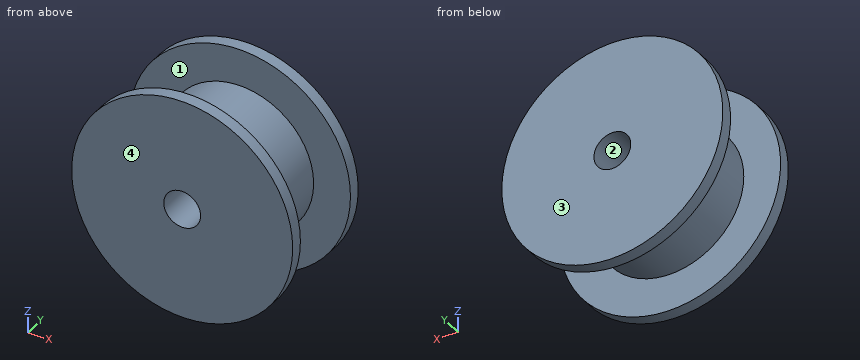
from build123d import *

# Parameters (mm, degrees)
SKETCH_1_R          = 9
EXTRUDE_1_DEPTH     = 1
SKETCH_2_R          = 6
EXTRUDE_2_DEPTH     = 6.5
SKETCH_3_R          = 9
EXTRUDE_3_DEPTH     = 1
SKETCH_4_R          = 1.5
CUT_EXTRUDE_1_DEPTH = 9.5


with BuildPart() as part:
    # 草图1 → 凸台-拉伸1 (new body)
    with BuildSketch(Plane(origin=(0, 0, 0), x_dir=(1, 0, 0), z_dir=(0, 1, 0))):
        Circle(SKETCH_1_R)
    extrude(amount=EXTRUDE_1_DEPTH)

    # 草图2 → 凸台-拉伸2 (add)
    with BuildSketch(Plane(origin=(0, 1, 0), x_dir=(1, 0, 0), z_dir=(0, 1, 0))):
        Circle(SKETCH_2_R)
    extrude(amount=EXTRUDE_2_DEPTH)

    # 草图3 → 凸台-拉伸3 (add)
    with BuildSketch(Plane(origin=(0, 7.5, 0), x_dir=(1, 0, 0), z_dir=(0, 1, 0))):
        Circle(SKETCH_3_R)
    extrude(amount=EXTRUDE_3_DEPTH)

    # 草图4 → 切除-拉伸1 (cut, through all)
    with BuildSketch(Plane(origin=(0, 8.5, 0), x_dir=(1, 0, 0), z_dir=(0, 1, 0))):
        Circle(SKETCH_4_R)
    extrude(amount=-CUT_EXTRUDE_1_DEPTH, mode=Mode.SUBTRACT)


solid = part.part
Can you work these out from the model? Positions are in its coordinate system, mm. Face numbers are marked on the shaded views. Coordinates: 2 decimals unless noted, no trailing zeros. Loops run counter-clockwise (first coordinate to the right, second up) from the corner with the lowest first, then second, coordinate; pieces in that order, holes last. Notation, with made-up numbers: M 52.25,82 L 111.25,82 A18 ccw 111.25,116 Z; hole C 38,-22.5 d10. An arc over 180 degrees is marked long. Answer as CSV lines item,"result". Start each with the question number.
1. If I drill on probe 1 along Z at (x, y) = (0, 3.75); probe 2 along Y at (x, z) = (-7, 4.75), over which ranges is the centre line in solid material (lowest first)? Write a range as [from, to].
2. Suppose I cut it at A-A, the plane x = 0. List the corners of the cut face in (y, z) for me.
3. For pin 1 Ø1 at (x, y) = (3, 4) entering from -Z, with a flat end and sliding along its axis, tell me the tip position at first contact or that it passes through.
4. Suppose I cut it at B-B, the plane z = 0. List the corners of the cut face in (x, y) for me.
5. Thinking about a two-plate mould opening in Y: for the marked faces 1, 2, 3 and 4, which applies, +Y half, -Y half, draft (parallel to the pull), parting line (faces both ways), or undercut?
6. Suppose I cut it at D-D, the plane z = -4.5. List the corners of the cut face in (x, y) for me, plus the area to 3 significant figures.
7. Suppose I cut it at C-C, the plane y = 5.5. List the corners of the cut face in (x, z) for me.
Output:
1,probe 1,"z = [-6, -1.5], [1.5, 6]"
1,probe 2,"y = [0, 1], [7.5, 8.5]"
2,outline,"M 0,-9 L 1,-9 L 1,-6 L 7.5,-6 L 7.5,-9 L 8.5,-9 L 8.5,-1.5 L 0,-1.5 Z; M 0,1.5 L 8.5,1.5 L 8.5,9 L 7.5,9 L 7.5,6 L 1,6 L 1,9 L 0,9 Z"
3,pin 1,"stops at z = -5.45"
4,outline,"M -9,0 L -1.5,0 L -1.5,8.5 L -9,8.5 L -9,7.5 L -6,7.5 L -6,1 L -9,1 Z; M 1.5,0 L 9,0 L 9,1 L 6,1 L 6,7.5 L 9,7.5 L 9,8.5 L 1.5,8.5 Z"
5,face 1,"undercut"
5,face 2,"draft"
5,face 3,"+Y half"
5,face 4,"-Y half"
6,outline,"M -7.79,0 L 7.79,0 L 7.79,1 L 3.97,1 L 3.97,7.5 L 7.79,7.5 L 7.79,8.5 L -7.79,8.5 L -7.79,7.5 L -3.97,7.5 L -3.97,1 L -7.79,1 Z"
6,area,"82.8 mm^2"
7,outline,"C 0,0 d12; hole C 0,0 d3"
